```python
from build123d import *

# Parameters (mm, degrees)
PAD052_DEPTH            = 500
POCKET004_DEPTH         = 1.001
POCKET005_DEPTH         = 1.001
BODY053_PITCH_ANGLE     = -90
BODY053_PLACEMENT_ANGLE = -90


with BuildPart() as part:
    # Sketch061 → Pad052 (new body)
    with BuildSketch(Plane.XZ):
        Polygon((0, 0), (0, 9.5), (1, 9.5), (1, 0), (0.8, 0), (0.8, 9.3), (0.2, 9.3), (0.2, 0), align=None)
    extrude(amount=PAD052_DEPTH)

    # Sketch060 → Pocket004 (cut, through all)
    with BuildSketch(Plane.YZ):
        Polygon((0, 0), (0, 9.5), (-9.5, 0), align=None)
    extrude(amount=POCKET004_DEPTH, mode=Mode.SUBTRACT)

    # Sketch062 → Pocket005 (cut, through all)
    with BuildSketch(Plane.YZ):
        Polygon((-500, 0), (-490.5, 0), (-500, 9.5), align=None)
    extrude(amount=POCKET005_DEPTH, mode=Mode.SUBTRACT)


with BuildPart() as part_1:
    # Body053 pitch: moved
    add(part.part.rotate(Axis((0, 0, 0), (0, 1, 0)), BODY053_PITCH_ANGLE))


with BuildPart() as part_2:
    # Body053 placement: moved
    add(part_1.part.moved(Location((504.546315, -15.421231, 0))).rotate(Axis((504.546315, -15.421231, 0), (0, 0, 1)), BODY053_PLACEMENT_ANGLE))


solid = part_2.part
```
Input: part model. Units: mm. Frame: model coordinates. Round coordinates to 2 decimals unless told otherwise and drop trailing zeros. Loops run counter-clockwise (first coordinate to the right, second up) from the corner with the lowest first, then second, coordinate; pieces in that order, holes last. Notation, with made-up numbers: (-0.75, -26.75) -> (23.25, -26.75) arc R9 cw to (23.25, -11.75) -> close; hole circle Ø8 at (16.5, -34). An arc over 180 degrees is marked (long way). Use one line per item in the form item = value. Start each with the question number.
Item 1: Mould query, pull axis Z, two halves, no side actions, for faces 1 (the face through (258, -11, 1)), 2 (the face through (258, -11, 0.2)), 3 (the face through (258, -11, 0)). Classes: pulls with the +Z half, pulls with the -Z half, needs draft (parallel to the pull), parting line crosses it, or undercut.
Item 2: Section query A-A on y = -13.5. Return the cut outline in (x, z), then the cut area to 3 significant figures.
Item 3: Material intervals for L1, parallel to Z at x = 38.5, y = -8.25; L2, parallel to Y at x = 426, z = 0.75; L3, parallel to X at y = -15, z = 0.1, sorted ascending. Write a range as from..to.
Item 4: Section query B-B on x = 310. Return the cut outline in (y, z).
Item 5: Section query C-C on z = 0.6. Return the cut outline in (x, y), then the cut area to 4 significant figures.
Ans:
q1.face_1 = pulls with the +Z half
q1.face_2 = undercut
q1.face_3 = pulls with the -Z half
q2.outline = (12.13, 0) -> (496.97, 0) -> (496.97, 0.2) -> (12.13, 0.2) -> close; (12.13, 0.8) -> (496.97, 0.8) -> (496.97, 1) -> (12.13, 1) -> close
q2.area = 194 mm^2
q3.L1 = 0..0.2, 0.8..1
q3.L2 = -6.12..-5.92
q3.L3 = 13.63..495.47
q4.outline = (-15.42, 0) -> (-5.92, 0) -> (-5.92, 1) -> (-15.42, 1) -> (-15.42, 0.8) -> (-6.12, 0.8) -> (-6.12, 0.2) -> (-15.42, 0.2) -> close
q5.outline = (4.55, -5.92) -> (4.75, -6.12) -> (504.35, -6.12) -> (504.55, -5.92) -> close
q5.area = 100.0 mm^2
